Here's how the part is built. I have some questions about the finished solid (model axes, mm). A direction names the side the tool comes from. Coordinates: 2 decimals unless noted, no trailing zeros. Write each loop counter-clockwise with the first axis right and the second up, starting at its lowest first coordinate (ties: lowest second). Pieces come first, ordered by that corner, then holes.
Item 1: We'd pull the mould along Y, two halves only. Please class faces 1 (the face through (6.49, 35.445, 8.902)), 2 (the face through (26.05, -1, 9)), 3 (the face through (23.05, 0, 9)): +Y half, -Y half, draft (parallel to the pull), parting line (faces both ways), or undercut.
Item 2: I'm going to push flat-ended pins straight in: pin 1 Ø10 at (x, y) = (-1.5, 21) entering from +Z; pin 2 Ø8 at (y, z) = (27, 6) entering from -X; pin 3 Ø6.5 at (x, z) = (-0.5, 11.5) entering from +Y. Where does each tip first touch, or does it pass through?
Item 3: For faces 4 (the face through (-10.95, -1, 9)), 5 (the face through (14.62, -17.61, 7.5)), 6 (the face through (6, 23.7, 1)), which set-ups out of +Z, -Z, +X, -X, +Y, -Y let a thin tool reach every point of the face, with its end or its side?
Item 4: If I drill on line 1 (Y direction, x = 6.05, z = 1.95); line 2 (X direction, y = 4, z = 15), over which ranges is the centre line in solid material (lowest first)?
Item 5: If we section it at A-A (y = -11): Please give me the cut outline in (x, z), then the cut area to 3 significant figures.
Item 6: If we section it at B-B (z = 7.75): Please give me the cut outline in (x, y), then the cut area to 3 significant figures.
from build123d import *

# Parameters (mm, degrees)
F0_R     = 1
F1_DEPTH = 3
F2_DEPTH = 16
F3_R     = 2
F4_W     = 10
F4_H     = 10
F5_DEPTH = 3
F6_R     = 5


# Not quite as in the source:
# - a feature names something its author has since deleted; it is built from what else it names


with BuildPart() as f1:
    # F0 (on Top) → F1 (new body)
    with BuildSketch(Plane.XY):
        with BuildLine():
            Line((-10.95, 4.9143462471), (-10.95, 15.45))
            ThreePointArc((-10.95, 15.45), (6.05, 32.45), (23.05, 15.45))
            Line((23.05, 15.45), (23.05, 4.9143462471))
            ThreePointArc((23.05, 4.9143462471), (25.2853840617, 9.9727744249), (26.05, 15.45))
            ThreePointArc((26.05, 15.45), (6.05, 35.45), (-13.95, 15.45))
            ThreePointArc((-13.95, 15.45), (-13.1853840617, 9.9727744249), (-10.95, 4.9143462471))
        make_face()
        with BuildLine():
            Line((-10.95, -16.1332358822), (-10.95, 4.9143462471))
            ThreePointArc((-10.95, 4.9143462471), (-13.1853840617, 9.9727744249), (-13.95, 15.45))
            Line((-13.95, 15.45), (-13.95, -19.1332358822))
            Line((-13.95, -19.1332358822), (6.05, -19.1332358822))
            Line((6.05, -19.1332358822), (6.05, -16.1332358822))
            Line((6.05, -16.1332358822), (-10.95, -16.1332358822))
        make_face()
        with BuildLine():
            ThreePointArc((26.05, 15.45), (25.2853840617, 9.9727744249), (23.05, 4.9143462471))
            Line((23.05, 4.9143462471), (23.05, -16.1332358822))
            Line((23.05, -16.1332358822), (6.05, -16.1332358822))
            Line((6.05, -16.1332358822), (6.05, -19.1332358822))
            Line((6.05, -19.1332358822), (26.05, -19.1332358822))
            Line((26.05, -19.1332358822), (26.05, 15.45))
        make_face()
        with BuildLine():
            Line((0, 0), (0, 11.35))
            Line((0, 11.35), (-3, 11.35))
            Line((-3, 11.35), (-3, 1.0591174697))
            ThreePointArc((-3, 1.0591174697), (-1.5369696903, 0.2369171133), (0, -0.4370230062))
            Line((0, -0.4370230062), (0, 0))
        make_face()
        with BuildLine():
            Line((-3, -4.8), (-3, -2.3852880549))
            ThreePointArc((-3, -2.3852880549), (-7.4767065554, 0.7181226667), (-10.95, 4.9143462471))
            Line((-10.95, 4.9143462471), (-10.95, -16.1332358822))
            Line((-10.95, -16.1332358822), (6.05, -16.1332358822))
            Line((6.05, -16.1332358822), (6.05, -4.8))
            Line((6.05, -4.8), (-3, -4.8))
        make_face()
        with BuildLine():
            ThreePointArc((23.05, 4.9143462471), (19.5767065554, 0.7181226667), (15.1, -2.3852880549))
            Line((15.1, -2.3852880549), (15.1, -4.8))
            Line((15.1, -4.8), (6.05, -4.8))
            Line((6.05, -4.8), (6.05, -16.1332358822))
            Line((6.05, -16.1332358822), (23.05, -16.1332358822))
            Line((23.05, -16.1332358822), (23.05, 4.9143462471))
        make_face()
        with BuildLine():
            Line((-3, 1.0591174697), (-3, 11.35))
            Line((-3, 11.35), (-3, 27.5))
            Line((-3, 27.5), (15.1, 27.5))
            Line((15.1, 27.5), (15.1, 1.0591174697))
            ThreePointArc((15.1, 1.0591174697), (20.9303561785, 7.2295985499), (23.05, 15.45))
            ThreePointArc((23.05, 15.45), (6.05, 32.45), (-10.95, 15.45))
            ThreePointArc((-10.95, 15.45), (-8.8303561785, 7.2295985499), (-3, 1.0591174697))
        make_face()
        with BuildLine():
            ThreePointArc((23.05, 15.45), (20.9303561785, 7.2295985499), (15.1, 1.0591174697))
            Line((15.1, 1.0591174697), (15.1, -2.3852880549))
            ThreePointArc((15.1, -2.3852880549), (19.5767065554, 0.7181226667), (23.05, 4.9143462471))
            Line((23.05, 4.9143462471), (23.05, 15.45))
        make_face()
        with BuildLine():
            Line((-3, -2.3852880549), (-3, 1.0591174697))
            ThreePointArc((-3, 1.0591174697), (-8.8303561785, 7.2295985499), (-10.95, 15.45))
            Line((-10.95, 15.45), (-10.95, 4.9143462471))
            ThreePointArc((-10.95, 4.9143462471), (-7.4767065554, 0.7181226667), (-3, -2.3852880549))
        make_face()
        with BuildLine():
            Line((0, -1), (0, -0.4370230062))
            ThreePointArc((0, -0.4370230062), (-1.5369696903, 0.2369171133), (-3, 1.0591174697))
            Line((-3, 1.0591174697), (-3, -2.3852880549))
            ThreePointArc((-3, -2.3852880549), (1.3973535003, -4.0012950867), (6.05, -4.55))
            Line((6.05, -4.55), (6.05, -3.5))
            ThreePointArc((6.05, -3.5), (5.0618917373, -2.6537597518), (5.7461374375, -1.5472841226))
            ThreePointArc((5.7461374375, -1.5472841226), (3.7372080924, -1.3919415031), (1.7607692997, -1))
            Line((1.7607692997, -1), (0, -1))
        make_face()
        with BuildLine():
            ThreePointArc((6.05, -4.55), (1.3973535003, -4.0012950867), (-3, -2.3852880549))
            Line((-3, -2.3852880549), (-3, -4.8))
            Line((-3, -4.8), (6.05, -4.8))
            Line((6.05, -4.8), (6.05, -4.55))
        make_face()
        with BuildLine():
            Line((15.1, -4.8), (15.1, -2.3852880549))
            ThreePointArc((15.1, -2.3852880549), (10.7026464997, -4.0012950867), (6.05, -4.55))
            Line((6.05, -4.55), (6.05, -4.8))
            Line((6.05, -4.8), (15.1, -4.8))
        make_face()
        with BuildLine():
            ThreePointArc((15.1, 1.0591174697), (13.6369696903, 0.2369171133), (12.1, -0.4370230062))
            Line((12.1, -0.4370230062), (12.1, -1))
            Line((12.1, -1), (10.3392307003, -1))
            ThreePointArc((10.3392307003, -1), (8.3627919076, -1.3919415031), (6.3538625625, -1.5472841226))
            ThreePointArc((6.3538625625, -1.5472841226), (6.8574226163, -1.9100265101), (7.05, -2.5))
            ThreePointArc((7.05, -2.5), (6.7571067812, -3.2071067812), (6.05, -3.5))
            Line((6.05, -3.5), (6.05, -4.55))
            ThreePointArc((6.05, -4.55), (10.7026464997, -4.0012950867), (15.1, -2.3852880549))
            Line((15.1, -2.3852880549), (15.1, 1.0591174697))
        make_face()
        with BuildLine():
            Line((10.3392307003, -1), (6.05, -1))
            Line((6.05, -1), (6.05, -1.5))
            ThreePointArc((6.05, -1.5), (6.2037597518, -1.5118917373), (6.3538625625, -1.5472841226))
            ThreePointArc((6.3538625625, -1.5472841226), (8.3627919076, -1.3919415031), (10.3392307003, -1))
        make_face()
        with BuildLine():
            Line((6.05, -1.5), (6.05, -1))
            Line((6.05, -1), (1.7607692997, -1))
            ThreePointArc((1.7607692997, -1), (3.7372080924, -1.3919415031), (5.7461374375, -1.5472841226))
            ThreePointArc((5.7461374375, -1.5472841226), (5.8962402482, -1.5118917373), (6.05, -1.5))
        make_face()
        with BuildLine():
            Line((0, 11.35), (0, 22.7))
            Line((0, 22.7), (0, 23.7))
            Line((0, 23.7), (12.1, 23.7))
            Line((12.1, 23.7), (12.1, 22.7))
            Line((12.1, 22.7), (12.1, 0))
            Line((12.1, 0), (12.1, -0.4370230062))
            ThreePointArc((12.1, -0.4370230062), (13.6369696903, 0.2369171133), (15.1, 1.0591174697))
            Line((15.1, 1.0591174697), (15.1, 27.5))
            Line((15.1, 27.5), (-3, 27.5))
            Line((-3, 27.5), (-3, 11.35))
            Line((-3, 11.35), (0, 11.35))
        make_face()
        with Locations((6.05, 25.2)):
            Circle(F0_R, mode=Mode.SUBTRACT)
    extrude(amount=F1_DEPTH)

    # F0 (on Top) → F2 (join)
    with BuildSketch(Plane.XY):
        with BuildLine():
            Line((-10.95, -16.1332358822), (-10.95, 4.9143462471))
            ThreePointArc((-10.95, 4.9143462471), (-13.1853840617, 9.9727744249), (-13.95, 15.45))
            Line((-13.95, 15.45), (-13.95, -19.1332358822))
            Line((-13.95, -19.1332358822), (6.05, -19.1332358822))
            Line((6.05, -19.1332358822), (6.05, -16.1332358822))
            Line((6.05, -16.1332358822), (-10.95, -16.1332358822))
        make_face()
        with BuildLine():
            ThreePointArc((26.05, 15.45), (25.2853840617, 9.9727744249), (23.05, 4.9143462471))
            Line((23.05, 4.9143462471), (23.05, -16.1332358822))
            Line((23.05, -16.1332358822), (6.05, -16.1332358822))
            Line((6.05, -16.1332358822), (6.05, -19.1332358822))
            Line((6.05, -19.1332358822), (26.05, -19.1332358822))
            Line((26.05, -19.1332358822), (26.05, 15.45))
        make_face()
        with BuildLine():
            Line((-10.95, 4.9143462471), (-10.95, 15.45))
            ThreePointArc((-10.95, 15.45), (6.05, 32.45), (23.05, 15.45))
            Line((23.05, 15.45), (23.05, 4.9143462471))
            ThreePointArc((23.05, 4.9143462471), (25.2853840617, 9.9727744249), (26.05, 15.45))
            ThreePointArc((26.05, 15.45), (6.05, 35.45), (-13.95, 15.45))
            ThreePointArc((-13.95, 15.45), (-13.1853840617, 9.9727744249), (-10.95, 4.9143462471))
        make_face()
    extrude(amount=F2_DEPTH)

    # F3
    f3_edges = [f1.edges().sort_by_distance(p)[0] for p in [
        (26.05, -1.841618, 0),
        (-13.95, -1.841618, 0),
        (6.05, -19.133236, 0),
        (26.05, -19.133236, 8),
        (-13.95, -19.133236, 8),
    ]]
    fillet(f3_edges, radius=F3_R)

    # F4 (on face) → F5 (cut, through all)
    with BuildSketch(Plane.XZ.offset(19.1332358822)):
        with Locations((1.05, 11)):
            Rectangle(F4_W, F4_H)
        with Locations((11.05, 11)):
            Rectangle(F4_W, F4_H)
    extrude(amount=-F5_DEPTH, mode=Mode.SUBTRACT)

    # F6
    f6_edges = [f1.edges().sort_by_distance(p)[0] for p in [
        (-3.95, -17.633236, 6),
        (16.05, -17.633236, 6),
    ]]
    fillet(f6_edges, radius=F6_R)


solid = f1.part
Answer list:
1. face 1: +Y half
1. face 2: draft
1. face 3: undercut
2. pin 1: stops at z = 3
2. pin 2: stops at x = -12.47
2. pin 3: stops at y = 35.18
3. face 4: +Z
3. face 5: +Z, -Y
3. face 6: +Z, -Z
4. line 1: y = -19.13 to -3.5, -1.5 to -1, 23.7 to 24.2, 26.2 to 35.45
4. line 2: x = -13.95 to -10.95, 23.05 to 26.05
5. outline: (-13.95, 2) arc R2 ccw to (-11.95, 0) - (24.05, 0) arc R2 ccw to (26.05, 2) - (26.05, 16) - (23.05, 16) - (23.05, 3) - (-10.95, 3) - (-10.95, 16) - (-13.95, 16) - close
5. area: 196 mm2
6. outline: (-13.95, -17.13) arc R2 ccw to (-11.95, -19.13) - (-2.75, -19.13) - (-2.75, -16.13) - (-10.95, -16.13) - (-10.95, 15.45) arc R17 cw to (23.05, 15.45) - (23.05, -16.13) - (14.85, -16.13) - (14.85, -19.13) - (24.05, -19.13) arc R2 ccw to (26.05, -17.13) - (26.05, 15.45) arc R20 ccw to (-13.95, 15.45) - close
6. area: 429 mm2
